For this review, take the finished solid that the model builds, in its own axes (mm). Round coordinates to 2 decimals unless told otherwise and drop trailing zeros. Loops run counter-clockwise (first coordinate to the right, second up) from the corner with the lowest first, then second, coordinate; pieces in that order, holes last.
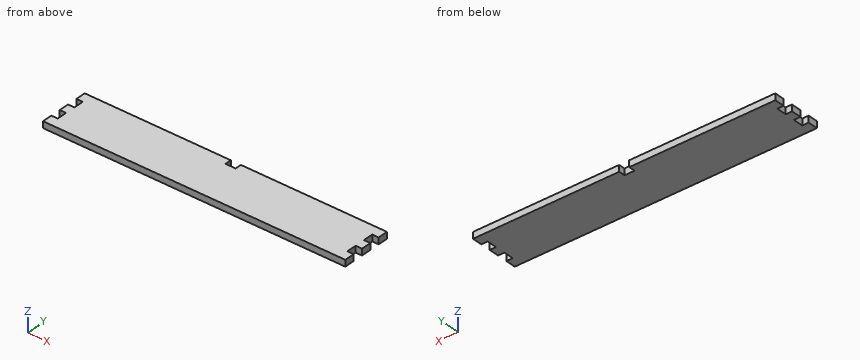
```python
from build123d import *

# Parameters (mm, degrees)
BOSS_EXTRUDE1_OUTLINE_W = 50
BOSS_EXTRUDE1_OUTLINE_H = 6.35
BOSS_EXTRUDE1_DEPTH     = 300
SKETCH1_W               = 10
SKETCH1_H               = 6.35
F_250_TOOTH_DEPTH       = 305.204409074
SKETCH5_W               = 6.35
SKETCH5_H               = 10
F_3T_CUT_DEPTH          = 305.204409074


# Read off the part's stored shape, not the designer's step: Boss-Extrude1
with BuildPart() as part:
    # Boss-Extrude1 outline → Boss-Extrude1 (new body)
    with BuildSketch(Plane.YZ):
        with Locations((25, 3.175)):
            Rectangle(BOSS_EXTRUDE1_OUTLINE_W, BOSS_EXTRUDE1_OUTLINE_H)
    extrude(amount=BOSS_EXTRUDE1_DEPTH)

    # Sketch1 → 250-tooth (cut, through all)
    with BuildSketch(Plane.XY.offset(6.35)):
        with Locations((150, 46.825)):
            Rectangle(SKETCH1_W, SKETCH1_H)
    extrude(amount=-F_250_TOOTH_DEPTH, mode=Mode.SUBTRACT)

    # Sketch5 → 3t_cut (cut, through all)
    with BuildSketch(Plane.XY.offset(6.35)):
        with Locations((3.175, 35)):
            Rectangle(SKETCH5_W, SKETCH5_H)
    f_3t_cut = extrude(amount=-F_3T_CUT_DEPTH, mode=Mode.SUBTRACT)

    # 3t_pattern: 3t_cut at 3 more places
    with Locations((0, -20, 0), (293.65, 0, 0), (293.65, -20, 0)):
        add(f_3t_cut, mode=Mode.SUBTRACT)


solid = part.part
```
(1) For L1, parallel to X at y = 36.5, z = 1.75; L2, parallel to X at y = 45.5, z = 0.75, list the stretches that pass through material, from the lowest coordinate up.
(2) Add section B-B (y = 13.5). Give the boundary of the cut face in (x, z), plus the area to 3 significant figures.
(3) Add section A-A (z = 1). Give the boundary of the cut face in (x, y).
Outcome:
1. L1: x = 6.35 to 293.65
1. L2: x = 0 to 145, 155 to 300
2. outline: (6.35, 0) - (293.65, 0) - (293.65, 6.35) - (6.35, 6.35) - close
2. area: 1,820 mm2
3. outline: (0, 0) - (300, 0) - (300, 10) - (293.65, 10) - (293.65, 20) - (300, 20) - (300, 30) - (293.65, 30) - (293.65, 40) - (300, 40) - (300, 50) - (155, 50) - (155, 43.65) - (145, 43.65) - (145, 50) - (0, 50) - (0, 40) - (6.35, 40) - (6.35, 30) - (0, 30) - (0, 20) - (6.35, 20) - (6.35, 10) - (0, 10) - close
